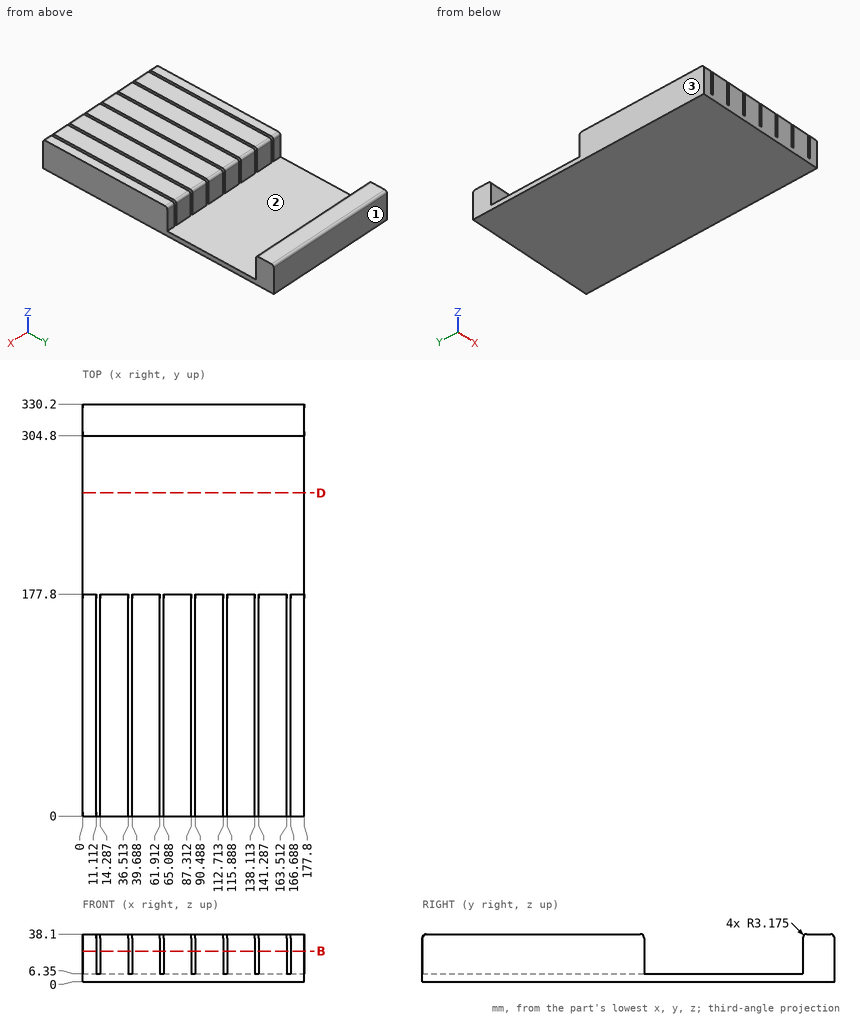
Can you work these out from the drawing? Everything is in mm from the part's minimum corner. Coordinates: 2 decimals unless noted, no trailing zeros. Loops run counter-clockwise (first coordinate to the right, second up) from the corner with the lowest first, then second, coordinate; pieces in that order, holes last.
1) Imagine slicing it at D-D (y = 259). List the corners of the cut face in (x, z) for me.
Reported:
outline: (0, 0) - (177.8, 0) - (177.8, 6.35) - (0, 6.35) - close
2) Please list where these lines run through material, in increasing order: line 1 along Y through (x, z) = (22, 32.5); line 2 along Z through (x, y) = (10.5, 191); line 3 along Y through (x, z) = (38.5, 26).
Reported:
line 1: y = 0 to 177.8, 304.8 to 330.2
line 2: z = 0 to 6.35
line 3: y = 304.8 to 330.2
3) Thinking about a two-plate mould opening in Y: for the marked faces 1, 2 and 3, which applies, released by +Y, released by -Y, zero draft, split by the parting line, or undercut?
Reported:
face 1: released by +Y
face 2: undercut
face 3: zero draft
4) Imagine slicing it at B-B (z = 24.5). State how many separate pieces and enclosed holes the cut face has, and give its area (3 significant figures).
Reported:
separate pieces: 9
enclosed holes: 0
area: 32,200 mm2
